from build123d import *

# Parameters (mm, degrees)
F1_DEPTH = 10.0203
F2_R     = 0.4699
F3_DEPTH = 25.4
F4_W     = 3.9624
F4_H     = 10.8966
F5_DEPTH = 25.4


with BuildPart() as f1:
    # F0 (on Top) → F1 (new body, symmetric)
    with BuildSketch(Plane.XY):
        with BuildLine():
            ThreePointArc((-12.9413, -1.3716), (-12.79251, -1.73081), (-12.4333, -1.8796))
            Line((-12.4333, -1.8796), (12.4333, -1.8796))
            ThreePointArc((12.4333, -1.8796), (12.79251, -1.73081), (12.9413, -1.3716))
            Line((12.9413, -1.3716), (12.9413, 1.3716))
            ThreePointArc((12.9413, 1.3716), (12.79251, 1.73081), (12.4333, 1.8796))
            Line((12.4333, 1.8796), (-12.4333, 1.8796))
            ThreePointArc((-12.4333, 1.8796), (-12.79251, 1.73081), (-12.9413, 1.3716))
            Line((-12.9413, 1.3716), (-12.9413, -1.3716))
        make_face()
    extrude(amount=F1_DEPTH, both=True)

    # F2 (on face) → F3 (cut)
    with BuildSketch(Plane.XY.offset(10.0203)):
        with Locations((11.6078, -0.6731)):
            Circle(F2_R)
        with Locations((-11.6078, -0.6731)):
            Circle(F2_R)
    extrude(amount=-F3_DEPTH, mode=Mode.SUBTRACT)

    # F4 (on face) → F5 (cut)
    with BuildSketch(Plane(origin=(0, 1.8796, 0), x_dir=(-1, 0, 0), z_dir=(0, 1, 0))):
        with Locations((-10.9601, 0)):
            Rectangle(F4_W, F4_H)
        with Locations((10.9601, 0)):
            Rectangle(F4_W, F4_H)
    extrude(amount=-F5_DEPTH, mode=Mode.SUBTRACT)


solid = f1.part
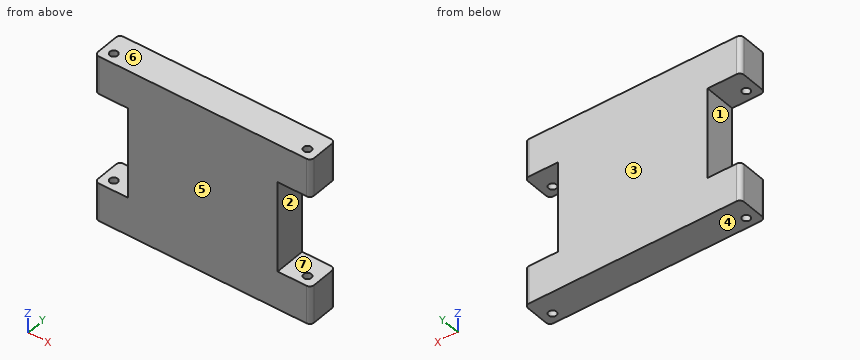
Model file for the job. Use its own axes, mm. Face numbers are marked on the shaded views. A direction names the side the tool comes from. Give positions to 0.01 mm unless a question says otherwise; leave off trailing zeros. Loops run counter-clockwise (first coordinate to the right, second up) from the corner with the lowest first, then second, coordinate; pieces in that order, holes last. Notation, with made-up numbers: (78, 48.25) -> (117, 48.25) arc R10 cw to (117, 60.25) -> close; hole circle Ø2 at (44, 73.5). An arc over 180 degrees is marked (long way). Use a Markdown table: item, result. Add a question column.
(1) Slice it at B-B on y = 0.85. List the corners of the cut face in (x, z).
(2) Mould opens along Z. For the marked faces 4, 5, 6 and 7 say: +Z half, -Z half, draft (parallel to the pull), parting line (faces both ways), or undercut.
(3) Tool access for the marked faces 1, 2 and 3: list every direction of +Z, -Z, +X, -X, +Y, -Y with a clear straight run to the whole face (end or side of a thin tool).
(4) Slice it at C-C on z = 9.25. List the corners of the cut face in (x, y).
(5) Wall check: line 1 along Z through (x, y) = (-10.75, -1.15); line 2 along X through (y, z) = (-0.8, -8.25); line 3 along X through (y, z) = (1.65, 2.25). Give the ranges that are in metal, low to high.
(6) Drop a flat-ended pin along its axis: pin 1 Ø1 at (y, z) = (-1, 0) entering from -X. Give the stop position or say it passes through.
(7) Slice it at D-D on z = -3.75. List the corners of the cut face in (x, y).
(8) Slice it at A-A on x = -9.5. List the corners of the cut face in (y, z).
Filled sheet:
| question | item | result |
|---|---|---|
| 1 | outline | (-12.94, -10.02) -> (12.94, -10.02) -> (12.94, -5.45) -> (8.98, -5.45) -> (8.98, 5.45) -> (12.94, 5.45) -> (12.94, 10.02) -> (-12.94, 10.02) -> (-12.94, 5.45) -> (-8.98, 5.45) -> (-8.98, -5.45) -> (-12.94, -5.45) -> close |
| 2 | face 4 | -Z half |
| 2 | face 5 | draft |
| 2 | face 6 | +Z half |
| 2 | face 7 | undercut |
| 3 | face 1 | -X, +Y, -Y |
| 3 | face 2 | +X, +Y, -Y |
| 3 | face 3 | +Z, -Z, +X, -X, +Y |
| 4 | outline | (-12.94, -1.37) arc R0.51 ccw to (-12.43, -1.88) -> (12.43, -1.88) arc R0.51 ccw to (12.94, -1.37) -> (12.94, 1.37) arc R0.51 ccw to (12.43, 1.88) -> (-12.43, 1.88) arc R0.51 ccw to (-12.94, 1.37) -> close; hole circle Ø0.94 at (-11.61, -0.67); hole circle Ø0.94 at (11.61, -0.67) |
| 5 | line 1 | -10.02 to -5.45, 5.45 to 10.02 |
| 5 | line 2 | -12.94 to -12.06, -11.16 to 11.16, 12.06 to 12.94 |
| 5 | line 3 | -8.98 to 8.98 |
| 6 | pin 1 | x = -8.98 |
| 7 | outline | (-8.98, -1.88) -> (8.98, -1.88) -> (8.98, 1.88) -> (-8.98, 1.88) -> close |
| 8 | outline | (-1.88, -10.02) -> (1.88, -10.02) -> (1.88, -5.45) -> (-1.88, -5.45) -> close; (-1.88, 5.45) -> (1.88, 5.45) -> (1.88, 10.02) -> (-1.88, 10.02) -> close |
